Build history of the part. All positions in model axes, mm. A direction names the side the tool comes from. Round coordinates to 2 decimals unless told otherwise and drop trailing zeros. Order: outer loops, then holes, each group sorted by start corner. A loop starts at its lowest first (then second) coordinate and runs counter-clockwise, first axis right, second up. Notation, with made-up numbers: (50, 27.5) -> (72, 27.5) arc R20 cw to (72, 65.5) -> close; hole circle Ø8 at (-35, 83). An arc over 180 degrees is marked (long way). Write item = value, one per line.
from build123d import *

# Parameters (mm, degrees)
BOARD3_R        = 1.5
EXTRUDE_4_DEPTH = 1.6


with BuildPart() as part:
    # Board3 → Бобышка-Вытянуть4 (new body)
    with BuildSketch(Plane.XY):
        with BuildLine():
            Line((12.870855766, 54), (44.970855766, 54))
            ThreePointArc((44.970855766, 54), (46.385069328, 53.414213562), (46.970855766, 52))
            Line((46.970855766, 52), (46.970855766, 49.700569912))
            ThreePointArc((46.970855766, 49.700569912), (46.677962547, 48.993463131), (45.970855766, 48.700569912))
            Line((45.970855766, 48.700569912), (39.93144499, 48.700569912))
            ThreePointArc((39.93144499, 48.700569912), (39.224338209, 48.407676693), (38.93144499, 47.700569912))
            Line((38.93144499, 47.700569912), (38.93144499, 46.541193448))
            ThreePointArc((38.93144499, 46.541193448), (39.224338209, 45.834086667), (39.93144499, 45.541193448))
            Line((39.93144499, 45.541193448), (45.970855766, 45.541193448))
            ThreePointArc((45.970855766, 45.541193448), (46.677962547, 45.248300229), (46.970855766, 44.541193448))
            Line((46.970855766, 44.541193448), (46.970855766, 40.140550153))
            ThreePointArc((46.970855766, 40.140550153), (46.677962547, 39.433443372), (45.970855766, 39.140550153))
            Line((45.970855766, 39.140550153), (39.728596312, 39.140550153))
            ThreePointArc((39.728596312, 39.140550153), (39.021489531, 38.847656935), (38.728596312, 38.140550153))
            Line((38.728596312, 38.140550153), (38.728596312, 16.029234453))
            ThreePointArc((38.728596312, 16.029234453), (39.021489531, 15.322127672), (39.728596312, 15.029234453))
            Line((39.728596312, 15.029234453), (45.970855766, 15.029234453))
            ThreePointArc((45.970855766, 15.029234453), (46.677962547, 14.736341234), (46.970855766, 14.029234453))
            Line((46.970855766, 14.029234453), (46.970855766, 10.412381856))
            ThreePointArc((46.970855766, 10.412381856), (46.385069328, 8.998168294), (44.970855766, 8.412381856))
            Line((44.970855766, 8.412381856), (12.870855766, 8.412381856))
            ThreePointArc((12.870855766, 8.412381856), (11.456642203, 8.998168294), (10.870855766, 10.412381856))
            Line((10.870855766, 10.412381856), (10.870855766, 21.919777804))
            ThreePointArc((10.870855766, 21.919777804), (11.163748985, 22.626884585), (11.870855766, 22.919777804))
            Line((11.870855766, 22.919777804), (15.023151862, 22.919777804))
            ThreePointArc((15.023151862, 22.919777804), (15.730258643, 23.212671023), (16.023151862, 23.919777804))
            Line((16.023151862, 23.919777804), (16.023151862, 38.110742779))
            ThreePointArc((16.023151862, 38.110742779), (15.730258643, 38.81784956), (15.023151862, 39.110742779))
            Line((15.023151862, 39.110742779), (11.870855766, 39.110742779))
            ThreePointArc((11.870855766, 39.110742779), (11.163748985, 39.403635998), (10.870855766, 40.110742779))
            Line((10.870855766, 40.110742779), (10.870855766, 52))
            ThreePointArc((10.870855766, 52), (11.456642203, 53.414213562), (12.870855766, 54))
        make_face()
        with Locations((13.670855766, 42.3)):
            Circle(BOARD3_R, mode=Mode.SUBTRACT)
        with Locations((44.270855766, 42.3)):
            Circle(BOARD3_R, mode=Mode.SUBTRACT)
        with Locations((13.670855766, 11.7)):
            Circle(BOARD3_R, mode=Mode.SUBTRACT)
        with Locations((44.270855766, 11.7)):
            Circle(BOARD3_R, mode=Mode.SUBTRACT)
    extrude(amount=EXTRUDE_4_DEPTH)


solid = part.part
Q1. Probe probe 1 along Y at (x, z) = (40.5, 0.4); probe 2 along X at (y, z) = (12.5, 1.05); probe 3 along X at (y, z) = (18.5, 0.45). List the from-to ranges inside material, lowest first.
Check values:
probe_1 = 8.41 to 15.03, 39.14 to 45.54, 48.7 to 54
probe_2 = 10.87 to 12.4, 14.94 to 43, 45.54 to 46.97
probe_3 = 10.87 to 38.73
Q2. Which spindle directions (+Z, -Z, +X, -X, +Y, -Y) get a long thin tool onto all of the face, cutting with end or side? Do faces 5 (the face through (46.401, 9.014, 0.789)), 6 (the face through (39.029, 38.855, 0.789)), 7 (the face through (11.156, 22.619, 0.789)). Say none if no direction does.
Check values:
face_5 = +Z, -Z, +X, -Y
face_6 = +Z, -Z, +X
face_7 = +Z, -Z, -X
Q3. Mould opens along X. For faces 1 (the face through (14.477, 43.565, 0.789)), 2 (the face through (46.67, 45.256, 0.789)), 3 (the face through (45.077, 43.565, 0.789)), 4 (the face through (29, 32, 0)) say: released by +X, released by -X, zero draft, split by the parting line, or undercut.
Check values:
face_1 = undercut
face_2 = released by +X
face_3 = undercut
face_4 = zero draft
Q4. Cut at C-C, the plane y = 36. List the corners of the cut face in (x, z), and give its area (3 significant figures).
Check values:
outline = (16.02, 0) -> (38.73, 0) -> (38.73, 1.6) -> (16.02, 1.6) -> close
area = 36.3 mm²
Q5. Cut at A-A, the plane y = 42.3. List the corners of the cut face in (x, z).
Check values:
outline = (10.87, 0) -> (12.17, 0) -> (12.17, 1.6) -> (10.87, 1.6) -> close; (15.17, 0) -> (42.77, 0) -> (42.77, 1.6) -> (15.17, 1.6) -> close; (45.77, 0) -> (46.97, 0) -> (46.97, 1.6) -> (45.77, 1.6) -> close
Q6. Cut at B-B, the plane z = 1.35. Give the number of separate pieces and of enclosed holes in the cut face, and give its area (3 significant figures).
Check values:
separate_pieces = 1
enclosed_holes = 4
area = 1,310 mm²
Q7. Flat gauge pin, fed straight in: pin 1 (0.6 mm diameter, centred on y = 47, z = 0.5, fed in from +X). Where does the tip first touch, or does it go through?
Check values:
pin_1 = 38.93
